The figure shows three views and two pictorial views of one solid part (mm, origin at its lowest corner). Answer the questions. Give positions to 0.01 mm unless a question says otherwise; leave off trailing zeros. Loops run counter-clockwise (first coordinate to the right, second up) from the corner with the lowest first, then second, coordinate; pieces in that order, holes last. Notation, with made-up numbers: (-29.5, 89.5) - (-6.5, 89.5) arc R19 cw to (-6.5, 114.5) - close; hole circle Ø2 at (-17, -13.5). An arc over 180 degrees is marked (long way). Write item = value, one per line.
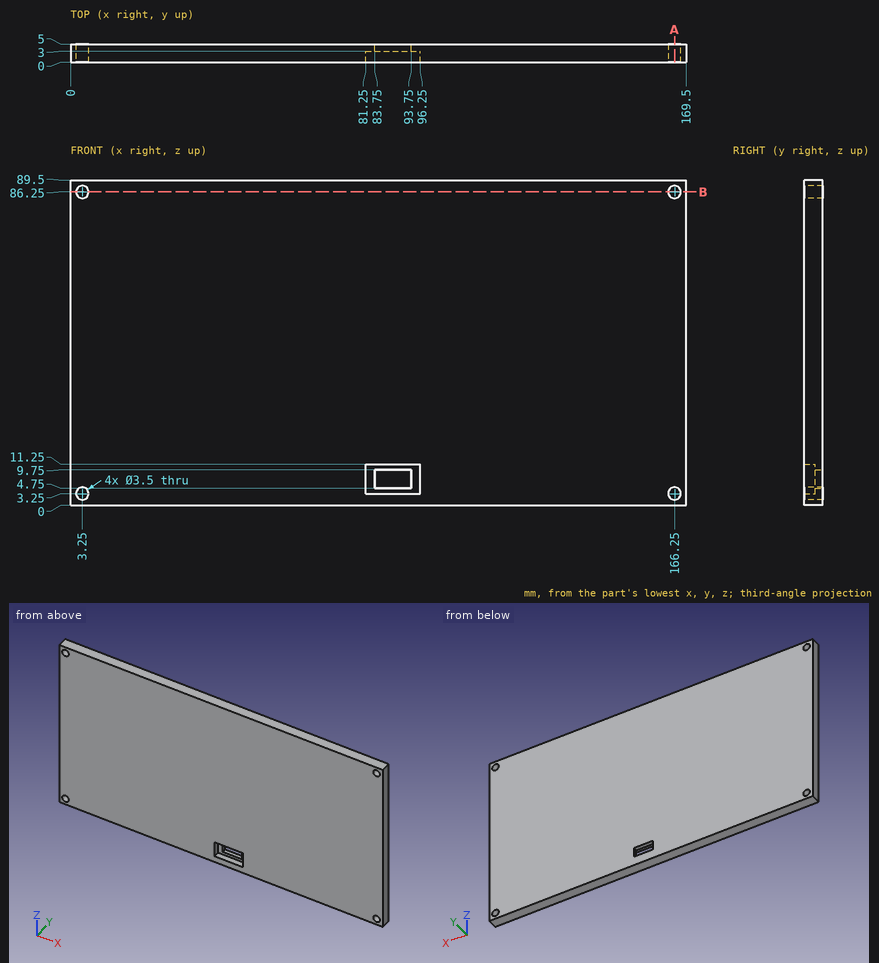
1) Find the intervals of material crossed by probe 1 along X at (y, z) = (3.45, 86.25); probe 2 along Z at (x, y) = (3.25, 1.9); probe 3 along Z at (x, y) = (84.5, 4.6), in increasing order.
Output:
probe_1 = 0 to 1.5, 5 to 164.5, 168 to 169.5
probe_2 = 0 to 1.5, 5 to 84.5, 88 to 89.5
probe_3 = 0 to 4.75, 9.75 to 89.5
2) Each of these flat-tipped pins is pushed along its axis until it touches: P1, Ø3, axis at x = 166.25, z = 3.25, coming from the +Y side; P2, Ø1, axis at y = 0.5, z = 14, coming from the -X side. Where does it stop, or does it pass through?
Output:
P1 = through
P2 = 0
3) A cutting plane is placed at B-B on z = 86.25. Determine the outline of the cut face in (x, y).
Output:
outline = (0, 0) - (1.5, 0) - (1.5, 5) - (0, 5) - close; (5, 0) - (164.5, 0) - (164.5, 5) - (5, 5) - close; (168, 0) - (169.5, 0) - (169.5, 5) - (168, 5) - close
4) A cutting plane is placed at A-A on x = 166.25. Determine the outline of the cut face in (y, z).
Output:
outline = (0, 0) - (5, 0) - (5, 1.5) - (0, 1.5) - close; (0, 5) - (5, 5) - (5, 84.5) - (0, 84.5) - close; (0, 88) - (5, 88) - (5, 89.5) - (0, 89.5) - close
